Model file for the job. Use its own axes, mm. Face numbers are marked on the shaded views. Round coordinates to 2 decimals unless told otherwise and drop trailing zeros. Loops run counter-clockwise (first coordinate to the right, second up) from the corner with the lowest first, then second, coordinate; pieces in that order, holes last. Notation, with made-up numbers: M 4.25,17 L 47.25,17 A26 cw 47.25,49 Z; hole C 48.5,44 d11. An arc over 180 degrees is marked long. Use a Markdown table: item, result. Add a question column.
Q1. Probe line 1 (Z direction, x = 8, y = 4); line 2 (Z direction, x = 6.25, y = 5); line 3 (Y direction, x = 3.25, z = 27.5). List the from-to ranges inside material, lowest first. Write a range as from..to.
Q2. Cut at C-C (z = 27.5). Give the cut face in (x, y).
Q3. Pin check, flat tips, straight feed: pin 1 (4 mm diameter, centred on x = 10, z = 9, fed in from -Y); pin 2 (1.5 mm diameter, centred on y = -5.5, z = 24, fed in from +X); pin 3 (2.5 mm diameter, centred on y = 4, z = 27.5, fed in from -X); pin 4 (4 mm diameter, centred on y = 4, z = 39.5, fed in from +X). Stop position of each tip, or through.
Q4. Cut at B-B (y = 4). Give the cut face in (x, z).
Q5. Cut at D-D (z = 7.5). Give the cut face in (x, y).
Q6. Cut at A-A (x = 8.5). Give the cut face in (y, z), plus the area to 3 significant figures.
Q7. Mould opens along Y. For the marked faces 1, 2 and 3 say: +Y half, -Y half, draft (parallel to the pull), parting line (faces both ways), or undercut.
from build123d import *

# Parameters (mm, degrees)
BOSS_EXTRU_1_DEPTH                             = 44.5
ESQUISSE2_W                                    = 15
ESQUISSE2_H                                    = 11.547005384
ENL_V_MAT_EXTRU_1_DEPTH                        = 46.105349392
ESQUISSE4_W                                    = 15
ESQUISSE4_H                                    = 11.547005384
ENL_V_MAT_EXTRU_3_DEPTH                        = 53.740449787
BOSS_EXTRU_4_DEPTH                             = 44.5
FRAISAGE_POUR_VIS_T_TE_FRAIS_E_M31_D           = 3.4
FRAISAGE_POUR_VIS_T_TE_FRAIS_E_M31_CSINK_D     = 6.3
FRAISAGE_POUR_VIS_T_TE_FRAIS_E_M31_CSINK_ANGLE = 90
R_P_TITION_LIN_AIRE1_COUNT                     = 2
R_P_TITION_LIN_AIRE1_PITCH                     = 12


with BuildPart() as part:
    # Esquisse1 → Boss.-Extru.1 (new body)
    with BuildSketch(Plane.XY):
        Polygon((0, 8), (5.773502692, 18), (9.226497308, 18), (15, 8), (15, 0), (0, 0), align=None)
    extrude(amount=BOSS_EXTRU_1_DEPTH)

    # Esquisse2 → Enlèv. mat.-Extru.1 (cut, through all)
    with BuildSketch(Plane(origin=(0, 21.269065234, 36.839101615), x_dir=(-1, 0, 0), z_dir=(0, 0.500000000000001, 0.866025403784438))):
        with Locations((-7.5, 9.548294078)):
            Rectangle(ESQUISSE2_W, ESQUISSE2_H)
    extrude(amount=ENL_V_MAT_EXTRU_1_DEPTH, mode=Mode.SUBTRACT)

    # Esquisse4 → Enlèv. mat.-Extru.3 (cut, through all)
    with BuildSketch(Plane(origin=(0, 2, -3.464101615), x_dir=(-1, 0, 0), z_dir=(0, 0.500000000000001, -0.866025403784438))):
        with Locations((-7.5, 12.701705922)):
            Rectangle(ESQUISSE4_W, ESQUISSE4_H)
    extrude(amount=ENL_V_MAT_EXTRU_3_DEPTH, mode=Mode.SUBTRACT)

    # Esquisse5 → Boss.-Extru.4 (add)
    with BuildSketch(Plane.XY):
        Polygon((0, -10), (5, -10), (15, 0), (0, 0), align=None)
    extrude(amount=BOSS_EXTRU_4_DEPTH)

    # Fraisage pour vis à tête fraisée M31 (through all)
    with Locations(Plane(origin=(15, 0, 0), x_dir=(0, 0, -1), z_dir=(1, 0, 0))):
        with Locations((-39.5, 4)):
            fraisage_pour_vis_t_te_frais_e_m31 = CounterSinkHole(FRAISAGE_POUR_VIS_T_TE_FRAIS_E_M31_D / 2, FRAISAGE_POUR_VIS_T_TE_FRAIS_E_M31_CSINK_D / 2, counter_sink_angle=FRAISAGE_POUR_VIS_T_TE_FRAIS_E_M31_CSINK_ANGLE)

    # Répétition linéaire1: Fraisage pour vis à tête fraisée M31 ×2
    with Locations(*[(0, 0, -i * R_P_TITION_LIN_AIRE1_PITCH) for i in range(1, R_P_TITION_LIN_AIRE1_COUNT)]):
        add(fraisage_pour_vis_t_te_frais_e_m31, mode=Mode.SUBTRACT)


solid = part.part
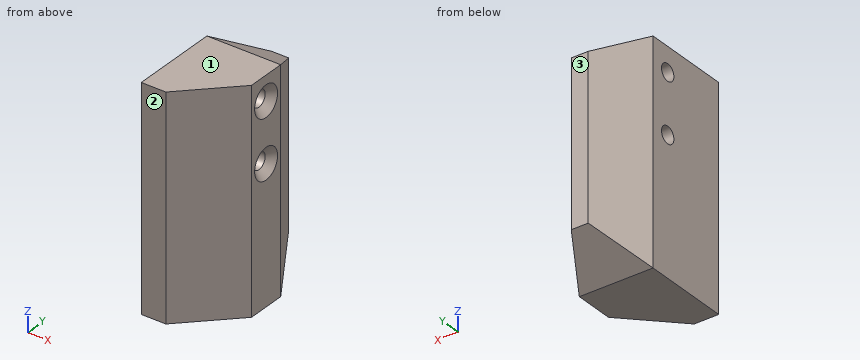
Checked values:
| question | item | result |
|---|---|---|
| 1 | line 1 | z = 0..25.8, 29.2..37.8, 41.2..44.5 |
| 1 | line 2 | z = 0..26.13, 28.87..38.13, 40.87..44.5 |
| 1 | line 3 | y = -10..2.3, 5.7..13.63 |
| 2 | outline | M 0,-10 L 5,-10 L 15,0 L 15,0.85 L 13.55,2.3 L 0,2.3 Z; M 0,5.7 L 13.55,5.7 L 15,7.15 L 15,8 L 9.23,18 L 5.77,18 L 0,8 Z |
| 3 | pin 1 | stops at y = -7 |
| 3 | pin 2 | stops at x = 10.25 |
| 3 | pin 3 | passes through |
| 3 | pin 4 | stops at x = 13.85 |
| 4 | outline | M 0,0 L 15,0 L 15,24.35 L 13.55,25.8 L 0,25.8 Z; M 0,29.2 L 13.55,29.2 L 15,30.65 L 15,36.35 L 13.55,37.8 L 0,37.8 Z; M 0,41.2 L 13.55,41.2 L 15,42.65 L 15,44.5 L 0,44.5 Z |
| 5 | outline | M 0,-10 L 5,-10 L 15,0 L 15,8 L 9.23,18 L 5.77,18 L 0,8 Z |
| 6 | outline | M -6.5,0 L 8,0 L 18,5.77 L 18,38.73 L 8,44.5 L -6.5,44.5 Z; hole C 4,27.5 d3.4; hole C 4,39.5 d3.4 |
| 6 | area | 1,010 mm^2 |
| 7 | face 1 | draft |
| 7 | face 2 | -Y half |
| 7 | face 3 | +Y half |
